Design review of the part built by this model. Coordinates are the model's own, in mm. A direction names the side the tool comes from. Give positions to 0.01 mm unless a question says otherwise; leave off trailing zeros. Loops run counter-clockwise (first coordinate to the right, second up) from the corner with the lowest first, then second, coordinate; pieces in that order, holes last.
from build123d import *

# Parameters (mm, degrees)
SKETCH1_W                    = 101.6
SKETCH1_H                    = 162.56
BOSS_EXTRUDE1_DEPTH          = 22.86
SKETCH2_W                    = 75
SKETCH2_H                    = 150.368
CUT_EXTRUDE1_DEPTH           = 10.7
SKETCH3_W                    = 72
SKETCH3_H                    = 11.000000098
LPATTERN1_COUNT              = 6
LPATTERN1_PITCH              = 25.622799961
M3_CLEARANCE_HOLE1_D         = 3.4
SKETCH10_R                   = 3.249999977
CUT_EXTRUDE2_DEPTH           = 5
SKETCH11_W                   = 11.43
SKETCH11_H                   = 162.56
CUT_EXTRUDE3_DEPTH           = 12.7
SKETCH12_W                   = 15.748
SKETCH12_H                   = 143.764
CUT_EXTRUDE4_DEPTH           = 6.35
SKETCH17_W                   = 63.5
SKETCH17_H                   = 6.096
CUT_EXTRUDE6_DEPTH           = 5.334
M3_START                     = 5.334
M3_CLEARANCE_HOLE2_OUTLINE_R = 1.7
M3_CLEARANCE_HOLE2_DEPTH     = 17.526
CUT_EXTRUDE8_DEPTH           = 5


# Read off the part's stored shape, not the designer's step: M3 Clearance Hole2
with BuildPart() as part:
    # Sketch1 → Boss-Extrude1 (new body)
    with BuildSketch(Plane(origin=(0, 0, 0), x_dir=(1, 0, 0), z_dir=(0, 1, 0))):
        Rectangle(SKETCH1_W, SKETCH1_H)
    extrude(amount=BOSS_EXTRUDE1_DEPTH)

    # Sketch2 → Cut-Extrude1 (cut)
    with BuildSketch(Plane.XZ):
        Rectangle(SKETCH2_W, SKETCH2_H)
    extrude(amount=-CUT_EXTRUDE1_DEPTH, mode=Mode.SUBTRACT)

    # Sketch3 → Cut-Revolve3 (revolve, cut)
    with BuildSketch(Plane.XZ.offset(-10.7)):
        with Locations((0, 69.556999951)):
            Rectangle(SKETCH3_W, SKETCH3_H)
    cut_revolve3 = revolve(axis=Axis((-36, 10.7, 64.056999902), (1, 0, 0)), mode=Mode.SUBTRACT)

    # LPattern1: Cut-Revolve3 ×6
    with Locations(*[(0, 0, -i * LPATTERN1_PITCH) for i in range(1, LPATTERN1_COUNT)]):
        add(cut_revolve3, mode=Mode.SUBTRACT)

    # M3 Clearance Hole1 (through all)
    with Locations(Plane(origin=(0, 22.86, 0), x_dir=(1, 0, 0), z_dir=(0, 1, 0))):
        with Locations((-16.51, 51.308), (-16.51, 25.654), (-16.51, 0), (-16.51, -25.654), (-16.51, -51.308), (16.51, -51.308), (16.51, -25.654), (16.51, 0), (16.51, 25.654), (16.51, 51.308)):
            Hole(M3_CLEARANCE_HOLE1_D / 2)

    # Sketch10 → Cut-Extrude2 (cut)
    with BuildSketch(Plane(origin=(0, 22.86, 0), x_dir=(1, 0, 0), z_dir=(0, 1, 0))):
        with Locations(Location((-16.51, 51.308, 0), (0, 0, 270))):
            Circle(SKETCH10_R)
        with Locations(Location((-16.51, 25.654, 0), (0, 0, 270))):
            Circle(SKETCH10_R)
        with Locations(Location((-16.51, 0, 0), (0, 0, 270))):
            Circle(SKETCH10_R)
        with Locations(Location((-16.51, -25.654, 0), (0, 0, 270))):
            Circle(SKETCH10_R)
        with Locations(Location((-16.51, -51.308, 0), (0, 0, 270))):
            Circle(SKETCH10_R)
        with Locations(Location((16.51, -51.308, 0), (0, 0, 90))):
            Circle(SKETCH10_R)
        with Locations(Location((16.51, -25.654, 0), (0, 0, 90))):
            Circle(SKETCH10_R)
        with Locations(Location((16.51, 0, 0), (0, 0, 90))):
            Circle(SKETCH10_R)
        with Locations(Location((16.51, 25.654, 0), (0, 0, 90))):
            Circle(SKETCH10_R)
        with Locations(Location((16.51, 51.308, 0), (0, 0, 90))):
            Circle(SKETCH10_R)
    extrude(amount=-CUT_EXTRUDE2_DEPTH, mode=Mode.SUBTRACT)

    # Sketch11 → Cut-Extrude3 (cut)
    with BuildSketch(Plane(origin=(0, 22.86, 0), x_dir=(1, 0, 0), z_dir=(0, 1, 0))):
        with Locations((-45.085, 0)):
            Rectangle(SKETCH11_W, SKETCH11_H)
        with Locations((45.085, 0)):
            Rectangle(SKETCH11_W, SKETCH11_H)
    extrude(amount=-CUT_EXTRUDE3_DEPTH, mode=Mode.SUBTRACT)

    # Sketch12 → Cut-Extrude4 (cut)
    with BuildSketch(Plane.XZ):
        with Locations((-42.926, 0)):
            Rectangle(SKETCH12_W, SKETCH12_H)
        with Locations((42.926, 0)):
            Rectangle(SKETCH12_W, SKETCH12_H)
    extrude(amount=-CUT_EXTRUDE4_DEPTH, mode=Mode.SUBTRACT)

    # Sketch17 → Cut-Extrude6 (cut)
    with BuildSketch(Plane.XZ):
        with Locations((0, -78.232)):
            Rectangle(SKETCH17_W, SKETCH17_H)
        with Locations((0, 78.232)):
            Rectangle(SKETCH17_W, SKETCH17_H)
    extrude(amount=-CUT_EXTRUDE6_DEPTH, mode=Mode.SUBTRACT)

    # M3 Clearance Hole2 outline → M3 Clearance Hole2 (cut)
    with BuildSketch(Plane(origin=(0, 0, 0), x_dir=(1, 0, 0), z_dir=(0, 1, 0)).offset(M3_START)):
        with Locations((16.51, -77.724)):
            Circle(M3_CLEARANCE_HOLE2_OUTLINE_R)
        with Locations((-16.51, -77.724)):
            Circle(M3_CLEARANCE_HOLE2_OUTLINE_R)
        with Locations((24.257, 77.724)):
            Circle(M3_CLEARANCE_HOLE2_OUTLINE_R)
        with Locations((-24.257, 77.724)):
            Circle(M3_CLEARANCE_HOLE2_OUTLINE_R)
    extrude(amount=M3_CLEARANCE_HOLE2_DEPTH, mode=Mode.SUBTRACT)

    # Sketch21 → Cut-Extrude8 (cut)
    with BuildSketch(Plane(origin=(0, 22.86, 0), x_dir=(1, 0, 0), z_dir=(0, 1, 0))):
        with BuildLine():
            Line((-27.559, 77.724), (-27.559, 81.28))
            Line((-27.559, 81.28), (-20.955, 81.28))
            Line((-20.955, 81.28), (-20.955, 77.724))
            ThreePointArc((-20.955, 77.724), (-24.257, 74.422), (-27.559, 77.724))
        make_face()
        with BuildLine():
            Line((20.955, 77.724), (20.955, 81.28))
            Line((20.955, 81.28), (27.559, 81.28))
            Line((27.559, 81.28), (27.559, 77.724))
            ThreePointArc((27.559, 77.724), (24.257, 74.422), (20.955, 77.724))
        make_face()
        with BuildLine():
            Line((-19.812, -77.724), (-19.812, -81.28))
            Line((-19.812, -81.28), (-13.208, -81.28))
            Line((-13.208, -81.28), (-13.208, -77.724))
            ThreePointArc((-13.208, -77.724), (-16.51, -74.422), (-19.812, -77.724))
        make_face()
        with BuildLine():
            Line((13.208, -77.724), (13.208, -81.28))
            Line((13.208, -81.28), (19.812, -81.28))
            Line((19.812, -81.28), (19.812, -77.724))
            ThreePointArc((19.812, -77.724), (16.51, -74.422), (13.208, -77.724))
        make_face()
    extrude(amount=-CUT_EXTRUDE8_DEPTH, mode=Mode.SUBTRACT)


solid = part.part
Q1. Insertion check: pin 1 (10.5 mm diameter, centred on x = -41, z = 7.5, fed in from -Y); pin 2 (3 mm diameter, centred on y = 10.5, z = -34.5, fed in from -X); pin 3 (3.5 mm diameter, centred on x = 43.5, z = -29.5, fed in from +Y); pin 4 (6.5 mm diameter, centred on y = 15.5, z = -31, fed in from -X). Each pin has a flat end and moves straight along its axis. Give the tip position at first contact, or say it passes through.
Results:
pin 1: stops at y = 6.35
pin 2: stops at x = -50.8
pin 3: stops at y = 10.16
pin 4: stops at x = -39.37
Q2. Tool access review of faces 4 (the face through (25.04, 17.86, -79.42)), 5 (the face through (0, 5.334, -78)), 6 (the face through (-39.37, 17, 1)): name each direction out of +Z, -Z, +X, -X, +Y, -Y from which nothing blocks a thin tool from reaching the whole face with its end or side.
Results:
face 4: -Z, +Y
face 5: +Z, -Z, -Y
face 6: +Z, -Z, -X, +Y
Q3. Take a section at B-B (x = -9). Give the boundary of the cut face in (y, z).
Results:
outline: (5.33, -81.28) - (22.86, -81.28) - (22.86, 81.28) - (5.33, 81.28) - (5.33, 75.18) - (10.7, 75.18) - (10.7, 75.06) arc R11 cw to (10.7, 53.06) - (10.7, 49.43) arc R11 cw to (10.7, 27.43) - (10.7, 23.81) arc R11 cw to (10.7, 1.81) - (10.7, -1.81) arc R11 cw to (10.7, -23.81) - (10.7, -27.43) arc R11 cw to (10.7, -49.43) - (10.7, -53.06) arc R11 cw to (10.7, -75.06) - (10.7, -75.18) - (5.33, -75.18) - close
Q4. Take a section at C-C (x = 16.51). Give the number of separate pieces and of enclosed holes in the cut face, plus the area to 3 significant figures.
Results:
separate pieces: 7
enclosed holes: 0
area: 541 mm2
Q5. Wall thickness on line 1 (X direction, y = 8.25, z = -32); line 2 (X direction, y = 12.25, z = -67.5); line 3 (X direction, y = 20.7, z = 0): over which ranges is each line inside the solid? List them lowest first.
Results:
line 1: x = -50.8 to -37.5, 37.5 to 50.8
line 2: x = -39.37 to -36, 36 to 39.37
line 3: x = -39.37 to -19.76, -13.26 to 13.26, 19.76 to 39.37
Q6. Draft analysis for pull direction Z (two halves, no side actions). For faces 1 (the face through (15, 17.86, 79)), 2 (the face through (-1, 11, 81.28)), 3 (the face through (18, 17.86, -53)), state which applies: pulls with the +Z half, pulls with the -Z half, needs draft (parallel to the pull), parting line crosses it, or undercut.
Results:
face 1: needs draft
face 2: pulls with the +Z half
face 3: undercut
Q7. Take a section at A-A (z = 0). Give the boundary of the cut face in (x, y).
Results:
outline: (-50.8, 6.35) - (-37.5, 6.35) - (-37.5, 10.7) - (-18.21, 10.7) - (-18.21, 17.86) - (-19.76, 17.86) - (-19.76, 22.86) - (-39.37, 22.86) - (-39.37, 10.16) - (-50.8, 10.16) - close; (-14.81, 10.7) - (14.81, 10.7) - (14.81, 17.86) - (13.26, 17.86) - (13.26, 22.86) - (-13.26, 22.86) - (-13.26, 17.86) - (-14.81, 17.86) - close; (18.21, 10.7) - (37.5, 10.7) - (37.5, 6.35) - (50.8, 6.35) - (50.8, 10.16) - (39.37, 10.16) - (39.37, 22.86) - (19.76, 22.86) - (19.76, 17.86) - (18.21, 17.86) - close
